Check sheet for the modelled part. Datum: model origin and axes. Units: mm. Face numbers are marked on the shaded views. A direction names the side the tool comes from. Coordinates: 2 decimals unless noted, no trailing zeros. Loops run counter-clockwise (first coordinate to the right, second up) from the corner with the lowest first, then second, coordinate; pieces in that order, holes last. Notation, with made-up numbers: M 41,-3.5 L 95,-3.5 A22 cw 95,27.5 Z; hole C -33,12 d11. An arc over 180 degrees is marked long. Use CSV: the item, a comma, the result in double quotes. Start each with the question number.
(1) Section check B-B on y = 45.5. Give the number of separate pieces and of enclosed holes in the cut face, and give its area (3 significant figures).
(2) Section check A-A on z = -40.5. Record the cut outline in (x, y) (3 decimals), and give its area (3 significant figures).
(3) Draft check along X on the marked faces 1, 2 and 3. Enter one of: pulls with the +X half, pulls with the -X half, needs draft (parallel to the pull), parting line crosses it, or undercut.
(4) Go/stop test with flat-tipped pins: pin 1 Ø1 at (x, z) = (46, -29) entering from -Y (3 decimals); pin 2 Ø5 at (x, z) = (46, 33.5) entering from -Y; pin 3 Ø1 at (x, z) = (-59, 15.5) entering from +Y (3 decimals). Record where each tip stops, or that it passes through.
(5) Set-up check for the marked faces 4 and 5: record each of +Z, -Z, +X, -X, +Y, -Y from which the full face is reachable in a straight line by a thin tool's end or side.
(6) Scan lines: line 1 (X direction, y = 59, z = -46) (3 decimals); line 2 (Y direction, x = -45, z = 33.5). Record each from-to range of solid material in increasing order.
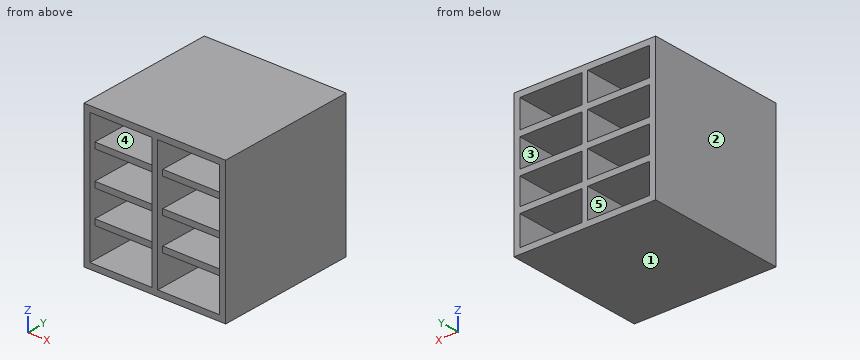
from build123d import *

# Parameters (mm, degrees)
F0_W     = 152.4
F0_H     = 152.4
F1_DEPTH = 76.2
F2_T     = -6.35
F3_W     = 6.35
F3_H     = 139.7
F4_DEPTH = 152.4
F5_W     = 139.7
F5_H     = 6.35
F6_DEPTH = 139.7
F7_DEPTH = 63.5
F8_W     = 152.4
F8_H     = 6.35
F9_DEPTH = 152.4


with BuildPart() as f1:
    # F0 (on Front) → F1 (new body, symmetric)
    with BuildSketch(Plane.XZ):
        Rectangle(F0_W, F0_H)
    extrude(amount=F1_DEPTH, both=True)

    # F2
    f2_openings = [f1.faces().sort_by_distance(p)[0] for p in [
        (0, -76.2, 0),
    ]]
    offset(amount=F2_T, openings=f2_openings)

    # F3 (on face) → F4 (join)
    with BuildSketch(Plane.XZ.offset(76.2)):
        Rectangle(F3_W, F3_H)
    extrude(amount=-F4_DEPTH)

    # F5 (on face) → F6 (join)
    with BuildSketch(Plane.YZ.offset(-69.85)):
        Rectangle(F5_W, F5_H)
        Polygon((-69.85, 33.3375), (69.85, 33.3375), (69.85, 36.5125), (69.85, 39.6875), (-69.85, 39.6875), (-69.85, 36.5125), align=None)
        with Locations((0, -34.925)):
            Rectangle(F5_W, F5_H)
    extrude(amount=F6_DEPTH)

    # F7 (cut, symmetric): faces of the model
    f7_faces = [f1.faces().sort_by_distance(p)[0] for p in [
        (-36.5125, 69.85, -53.975),
        (-36.5125, 69.85, -17.4625),
        (-36.5125, 69.85, 18.25625),
        (-36.5125, 69.85, 54.76875),
        (36.5125, 69.85, 54.76875),
        (36.5125, 69.85, 18.25625),
        (36.5125, 69.85, -17.4625),
        (36.5125, 69.85, -53.975),
    ]]
    extrude(f7_faces, amount=F7_DEPTH, both=True, mode=Mode.SUBTRACT)

    # F8 (on face) → F9 (join)
    with BuildSketch(Plane.XY.offset(76.2)):
        Rectangle(F8_W, F8_H)
    extrude(amount=-F9_DEPTH)


solid = f1.part
Outcome:
1,separate pieces,"1"
1,enclosed holes,"8"
1,area,"7,140 mm²"
2,outline,"M -76.2,-76.2 L -69.85,-76.2 L -69.85,-3.175 L -3.175,-3.175 L -3.175,-76.2 L 3.175,-76.2 L 3.175,-3.175 L 69.85,-3.175 L 69.85,-76.2 L 76.2,-76.2 L 76.2,76.2 L 69.85,76.2 L 69.85,3.175 L 3.175,3.175 L 3.175,76.2 L -3.175,76.2 L -3.175,3.175 L -69.85,3.175 L -69.85,76.2 L -76.2,76.2 Z"
2,area,"3,750 mm²"
3,face 1,"needs draft"
3,face 2,"pulls with the -X half"
3,face 3,"undercut"
4,pin 1,"stops at y = -3.175"
4,pin 2,"stops at y = -69.85"
4,pin 3,"stops at y = 3.175"
5,face 4,"-Y"
5,face 5,"+Y"
6,line 1,"x = -76.2 to -69.85, -3.175 to 3.175, 69.85 to 76.2"
6,line 2,"y = -69.85 to 76.2"
